Input: part model. Units: mm. Frame: model coordinates. Give positions to 0.01 mm unless a question says otherwise; leave off trailing zeros. Write each loop counter-clockwise with the first axis right and the second up, starting at its lowest first coordinate (ties: lowest second). Pieces come first, ordered by that corner, then holes. Notation, with made-up numbers: (-4, 59) -> (8, 59) arc R27 ccw to (8, 92) -> close; hole circle Ø1 at (15.25, -25.75). An arc over 180 degrees is marked (long way). Return JSON: item names as keys, results as strings. Group by question number.
Item 1: Line query: line 1 (X direction, y = 1.95, z = -12.7); line 2 (X direction, y = 1.1, z = -88.9); line 3 (Z direction, x = -50.5, y = 2.1). Output: solid intervals per line, ascending. Write a range as [from, to].
Item 2: Pin query (flat end, axial travel): P1, Ø1.5, axis at y = 1, z = -40, coming from the -X side. Return the tip coordinate at first contact, or that it passes through.
Item 3: Section C-C, the plane z = -88.9. Return loops of the section in (x, y).
Item 4: Section A-A, the plane z = -12.7. Return loops of the section in (x, y).
Item 5: Section B-B, the plane y = 1.65. Count the separate pieces of the cut face and the enclosed holes in it, then the cut area to 3 significant figures.
Item 6: Section D-D, the plane x = -25.4. Return loops of the section in (y, z).
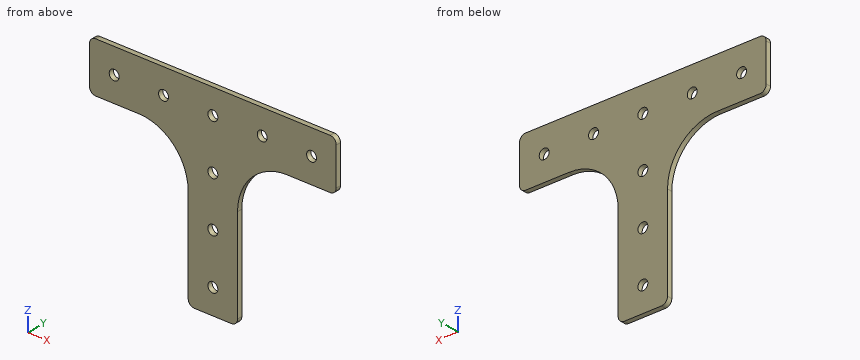
from build123d import *

# Parameters (mm, degrees)
BOSS_EXTRUDE1_DEPTH        = 2.54
FILLET1_R                  = 3.175
F_7_0_201_DIAMETER_HOLE1_D = 5.1054
FILLET2_R                  = 25.4


with BuildPart() as part:
    # Sketch1 → Boss-Extrude1 (new body)
    with BuildSketch(Plane(origin=(0, 0, 0), x_dir=(1, 0, 0), z_dir=(0, 1, 0))):
        Polygon((-63.5, 0), (63.5, 0), (63.5, 25.4), (12.7, 25.4), (12.7, 101.6), (-12.7, 101.6), (-12.7, 25.4), (-63.5, 25.4), align=None)
    extrude(amount=BOSS_EXTRUDE1_DEPTH)

    # Fillet1
    fillet1_edges = [part.edges().sort_by_distance(p)[0] for p in [
        (-12.7, 1.27, -101.6),
        (12.7, 1.27, -101.6),
        (63.5, 1.27, -25.4),
        (63.5, 1.27, 0),
        (-63.5, 1.27, 0),
        (-63.5, 1.27, -25.4),
    ]]
    fillet(fillet1_edges, radius=FILLET1_R)

    # #7 (0.201) Diameter Hole1 (through all)
    with Locations(Plane(origin=(0, 2.54, 0), x_dir=(1, 0, 0), z_dir=(0, 1, 0))):
        with Locations((0, 12.7), (25.4, 12.7), (50.8, 12.7), (-25.4, 12.7), (-50.8, 12.7), (0, 38.1), (0, 63.5), (0, 88.9)):
            Hole(F_7_0_201_DIAMETER_HOLE1_D / 2)

    # Fillet2
    fillet2_edges = [part.edges().sort_by_distance(p)[0] for p in [
        (12.7, 1.27, -25.4),
        (-12.7, 1.27, -25.4),
    ]]
    fillet(fillet2_edges, radius=FILLET2_R)


solid = part.part
Answer below:
{
 "1": {"line 1": "x = [-63.5, -53.35], [-48.25, -27.95], [-22.85, -2.55], [2.55, 22.85], [27.95, 48.25], [53.35, 63.5]", "line 2": "x = [-12.7, -2.55], [2.55, 12.7]", "line 3": "z = [-25.4, -15.24], [-10.16, 0]"},
 "2": {"P1": "stops at x = -15.48"},
 "3": {"outline": "(-12.7, 0) -> (-2.55, 0) -> (-2.55, 2.54) -> (-12.7, 2.54) -> close; (2.55, 0) -> (12.7, 0) -> (12.7, 2.54) -> (2.55, 2.54) -> close"},
 "4": {"outline": "(-63.5, 0) -> (-53.35, 0) -> (-53.35, 2.54) -> (-63.5, 2.54) -> close; (-48.25, 0) -> (-27.95, 0) -> (-27.95, 2.54) -> (-48.25, 2.54) -> close; (-22.85, 0) -> (-2.55, 0) -> (-2.55, 2.54) -> (-22.85, 2.54) -> close; (2.55, 0) -> (22.85, 0) -> (22.85, 2.54) -> (2.55, 2.54) -> close; (27.95, 0) -> (48.25, 0) -> (48.25, 2.54) -> (27.95, 2.54) -> close; (53.35, 0) -> (63.5, 0) -> (63.5, 2.54) -> (53.35, 2.54) -> close"},
 "5": {"separate pieces": "1", "enclosed holes": "8", "area": "5,260 mm2"},
 "6": {"outline": "(0, -28.8) -> (2.54, -28.8) -> (2.54, -15.25) -> (0, -15.25) -> close; (0, -10.15) -> (2.54, -10.15) -> (2.54, 0) -> (0, 0) -> close"}
}
